Read the model definition and answer for the solid it produces. Units are mm, in the model's axes. A direction names the side the tool comes from. Coordinates: 2 decimals unless noted, no trailing zeros. Order: outer loops, then holes, each group sorted by start corner. A loop starts at its lowest first (then second) coordinate and runs counter-clockwise, first axis right, second up. Notation, with made-up numbers: (70.5, 21.25) - (81.5, 21.25) arc R38 cw to (81.5, 60.25) - close; hole circle Ø7 at (23, 19.25). An arc over 180 degrees is marked (long way). Use one line per item in the form item = value.
Autodesk Inventor part; units mm, degrees
ref_plane "YZ Plane" through (0, 0, 0) normal (1, 0, 0) x (0, 1, 0)
ref_plane "XZ Plane" through (0, 0, 0) normal (0, 1, 0) x (-1, 0, 0)
ref_plane "XY Plane" through (0, 0, 0) normal (0, 0, 1) x (1, 0, 0)
sketch "スケッチ1" plane through (0, 0, 0) normal (0, 0, 1) x (1, 0, 0)
  line L0 (-5, 5) -> (5, 5)
  line L1 (5, 5) -> (5, -5)
  line L2 (5, -5) -> (-5, -5)
  line L3 (-5, -5) -> (-5, 5)
  line L4 (-5, 5) -> (5, -5) construction
  line L5 (5, 5) -> (-5, -5) construction
  line L6 (-4, 4) -> (4, 4)
  line L7 (4, 4) -> (4, -4)
  line L8 (4, -4) -> (-4, -4)
  line L9 (-4, -4) -> (-4, 4)
  line L10 (-4, 4) -> (4, -4) construction
  line L11 (4, 4) -> (-4, -4) construction
  point P0 (0, 0)
  dimension "d0" = 10
  dimension "d1" = 10
  dimension "d2" = 8
extrude "押し出し1" add sketch "スケッチ1" along normal blind 28
sketch "スケッチ2" plane through (-5, 5, 0) normal (0, 1, 0) x (1, 0, 0)
  circle A0 centre (5, -7) radius 1.4
  line L0 (0, 0) -> (0, -28)
  line L1 (0, -14) -> (10, -14)
  line L2 (10, 0) -> (10, -28)
  circle A1 centre (5, -21) radius 1.4
  point P0 (5, 0)
extrude "押し出し2" cut sketch "スケッチ2" against normal through all
properties part number "position_setter_bar" material "アルミニウム 6061"
(1) The mould has two halves that part along Z. Classify faces 3 (the flat face through (0, 5, 14)), 4 (the cylindrical face through (-0.303, 4.507, 22.367)), 5 (the flat face through (-4.5, 0.1, 28)): +Z half, -Z half, draft (parallel to the pull), parting line (faces both ways), or undercut.
Answer list:
face_3 = draft
face_4 = undercut
face_5 = +Z half
(2) Which of the six approach directions +Z, -Z, +X, -X, +Y, -Y give full straight-line access (tool end or side, diameter ignored) to faces 1 (the cylindrical face through (-0.303, -4.493, 22.367)), 2 (the flat face through (0, -4, 14))?
Answer list:
face_1 = +Y, -Y
face_2 = +Z, -Z
(3) Straight lines are drawn through the part: L1, parallel to Z at x = 0, y = -4.35; L2, parallel to Y at x = 3, z = 25.5; L3, parallel to X at y = 4.45, z = 7. For each, find the intervals that lie inside material, in ascending order.
Answer list:
L1 = 0 to 5.6, 8.4 to 19.6, 22.4 to 28
L2 = -5 to -4, 4 to 5
L3 = -5 to -1.4, 1.4 to 5
(4) Section A-A, the plane z = 9.75 is taken. Write down the section's boundary in (x, y), then the cut area to 3 significant figures.
Answer list:
outline = (-5, -5) - (5, -5) - (5, 5) - (-5, 5) - close; hole (-4, -4) - (4, -4) - (4, 4) - (-4, 4) - close
area = 36.0 mm2
(5) Section B-B, the plane x = 3.25 is taken. Write down the section's boundary in (y, z), then the cut area to 3 significant figures.
Answer list:
outline = (-5, 0) - (-4, 0) - (-4, 28) - (-5, 28) - close; (4, 0) - (5, 0) - (5, 28) - (4, 28) - close
area = 56.0 mm2
(6) Section C-C, the plane z = 21 is taken. Write down the section's boundary in (x, y), then the cut area to 3 significant figures.
Answer list:
outline = (-5, -5) - (-1.4, -5) - (-1.4, -4) - (-4, -4) - (-4, 4) - (-1.4, 4) - (-1.4, 5) - (-5, 5) - close; (1.4, -5) - (5, -5) - (5, 5) - (1.4, 5) - (1.4, 4) - (4, 4) - (4, -4) - (1.4, -4) - close
area = 30.4 mm2
